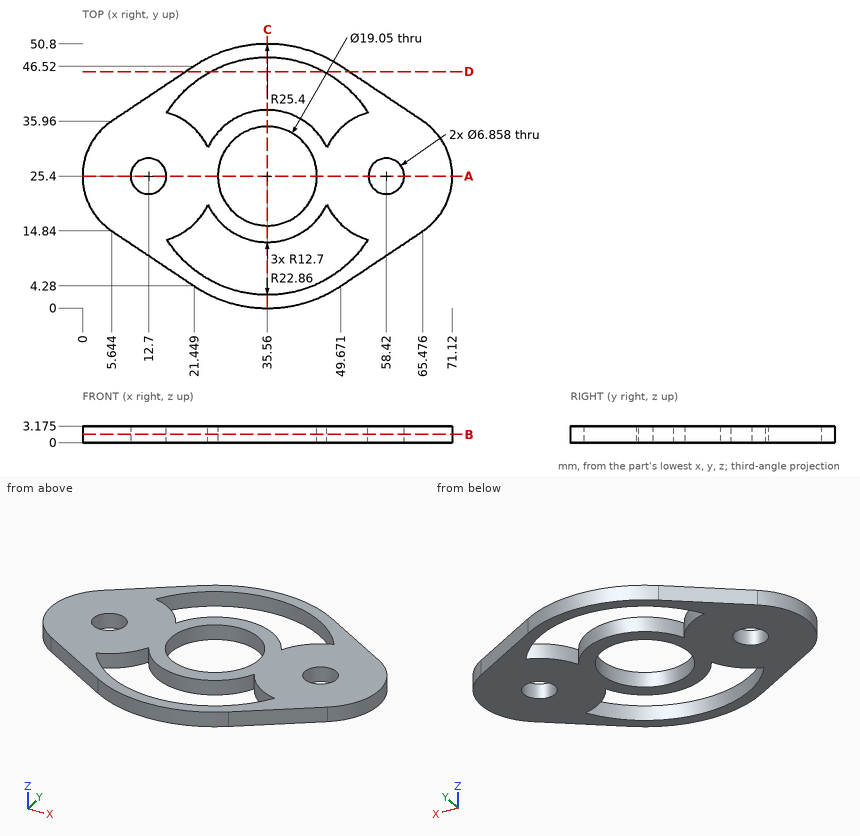
Design review of the part shown in the three views and the two pictorial views. Dimensions are in mm from the part's minimum x, y and z. Round coordinates to 2 decimals unless told otherwise and drop trailing zeros. Loops run counter-clockwise (first coordinate to the right, second up) from the corner with the lowest first, then second, coordinate; pieces in that order, holes last. Notation, with made-up numbers: (28.25, 56) -> (68.25, 56) arc R28 ccw to (68.25, 90) -> close; hole circle Ø6 at (-36, 54.25). An arc over 180 degrees is marked (long way). Answer as a JSON object with one key per item and string values. Group by question number.
1) We need section B-B on z = 1.6. Give the number of separate pieces and of enclosed holes in the cut face, then the cut area to 3 significant figures.
2) For line 1 (X direction, y = 33, z = 2.95) (1 decimal); line 2 (X direction, y = 18, z = 2.7) (1 decimal); line 3 (Y direction, x = 36.5, z = 1.05) (1 decimal), list the stretches that pass through material, from the lowest coordinate up. Write a range as [from, to].
3) For pin 1 Ø4 at (x, y) = (12.7, 25.4) entering from -Z; pin 2 Ø1.5 at (y, z) = (10.5, 1) entering from -X; pin 3 Ø1 at (y, z) = (40, 1.5) entering from +X (1 decimal), all flat-tipped, find the tip position at first contact; note any pin that passes through.
4) We need section C-C on x = 35.56. Write out the cut boundary in (y, z) (1 decimal).
5) We need section A-A on y = 25.4. Write out the cut boundary in (x, z) (1 decimal).
6) We need section D-D on y = 45.5. Write out the cut boundary in (x, z) (1 decimal).
Result set:
{
 "1": {"separate pieces": "1", "enclosed holes": "5", "area": "1,440 mm²"},
 "2": {"line 1": "[2.5, 22.9], [25.4, 29.8], [41.3, 45.7], [48.2, 68.6]", "line 2": "[2.4, 23], [25.2, 29.6], [41.6, 45.9], [48.1, 68.7]", "line 3": "[0, 2.6], [12.7, 15.9], [34.9, 38.1], [48.2, 50.8]"},
 "3": {"pin 1": "through", "pin 2": "x = 11.02", "pin 3": "x = 60.2"},
 "4": {"outline": "(0, 0) -> (2.5, 0) -> (2.5, 3.2) -> (0, 3.2) -> close; (12.7, 0) -> (15.9, 0) -> (15.9, 3.2) -> (12.7, 3.2) -> close; (34.9, 0) -> (38.1, 0) -> (38.1, 3.2) -> (34.9, 3.2) -> close; (48.3, 0) -> (50.8, 0) -> (50.8, 3.2) -> (48.3, 3.2) -> close"},
 "5": {"outline": "(0, 0) -> (9.3, 0) -> (9.3, 3.2) -> (0, 3.2) -> close; (16.1, 0) -> (26, 0) -> (26, 3.2) -> (16.1, 3.2) -> close; (45.1, 0) -> (55, 0) -> (55, 3.2) -> (45.1, 3.2) -> close; (61.8, 0) -> (71.1, 0) -> (71.1, 3.2) -> (61.8, 3.2) -> close"},
 "6": {"outline": "(19.9, 0) -> (24.7, 0) -> (24.7, 3.2) -> (19.9, 3.2) -> close; (46.4, 0) -> (51.2, 0) -> (51.2, 3.2) -> (46.4, 3.2) -> close"}
}
